Design review of the part built by this model. Coordinates are the model's own, in mm. A direction names the side the tool comes from. Coordinates: 2 decimals unless noted, no trailing zeros. Order: outer loops, then holes, each group sorted by start corner. A loop starts at its lowest first (then second) coordinate and runs counter-clockwise, first axis right, second up. Notation, with made-up numbers: M 28,59.5 L 77,59.5 A18 ccw 77,70.5 Z; hole C 74,-23 d7. An arc over 180 degrees is marked long. Answer as a JSON object with one key per item and string values.
from build123d import *

# Parameters (mm, degrees)
SKETCH3_R           = 12.7
BOSS_EXTRUDE1_DEPTH = 381
SKETCH4_W           = 50.8
SKETCH4_H           = 50.8
BOSS_EXTRUDE2_DEPTH = 25.4
SKETCH5_W           = 50.8
SKETCH5_H           = 50.8
BOSS_EXTRUDE3_DEPTH = 25.4
SKETCH6_R           = 1.016
SKETCH6_R_2         = 0.9921875
CUT_EXTRUDE1_DEPTH  = 411.349558304


with BuildPart() as part:
    # Sketch3 → Boss-Extrude1 (new body)
    with BuildSketch(Plane.XY):
        Circle(SKETCH3_R)
    extrude(amount=BOSS_EXTRUDE1_DEPTH)

    # Sketch4 → Boss-Extrude2 (add, symmetric)
    with BuildSketch(Plane(origin=(0, 0, 0), x_dir=(-1, 0, 0), z_dir=(0, 0, -1))):
        Rectangle(SKETCH4_W, SKETCH4_H)
    extrude(amount=BOSS_EXTRUDE2_DEPTH, both=True)

    # Sketch5 → Boss-Extrude3 (add, symmetric)
    with BuildSketch(Plane.XY.offset(381)):
        Rectangle(SKETCH5_W, SKETCH5_H)
    extrude(amount=BOSS_EXTRUDE3_DEPTH, both=True)

    # Sketch6 → Cut-Extrude1 (cut, through all)
    with BuildSketch(Plane(origin=(0, 25.4, 0), x_dir=(1, 0, 0), z_dir=(0, 1, 0))):
        with Locations(Location((0, -381, 0), (0, 0, 270))):
            Circle(SKETCH6_R)
        with Locations(Location((0, 0, 0), (0, 0, 270))):
            Circle(SKETCH6_R_2)
    extrude(amount=-CUT_EXTRUDE1_DEPTH, mode=Mode.SUBTRACT)


solid = part.part
1) Add section B-B (z = 326). State the section outline as (x, y) points, and give its area (3 significant figures).
Taken from the geometry:
{"outline": "C 0,0 d25.4", "area": "507 mm2"}
2) Add section A-A (y = 0). State the section outline as (x, z) points, and give its area (3 significant figures).
Taken from the geometry:
{"outline": "M -25.4,-25.4 L 25.4,-25.4 L 25.4,25.4 L 12.7,25.4 L 12.7,355.6 L 25.4,355.6 L 25.4,406.4 L -25.4,406.4 L -25.4,355.6 L -12.7,355.6 L -12.7,25.4 L -25.4,25.4 Z; hole C 0,381 d2.03; hole C 0,0 d1.98", "area": "13,500 mm2"}
3) To check wall thickness, follow L1, parallel to Z at x = -3, y = 17.5; L2, parallel to X at y = 9, z = 381; L3, parallel to Y at x = -0.5, z = 234. State the ranges of each line that lie inside material, in increasing order.
Taken from the geometry:
{"L1": "z = -25.4 to 25.4, 355.6 to 406.4", "L2": "x = -25.4 to -1.02, 1.02 to 25.4", "L3": "y = -12.69 to 12.69"}
4) Add section C-C (x = 7.5). State the section outline as (y, z) points.
Taken from the geometry:
{"outline": "M -25.4,-25.4 L 25.4,-25.4 L 25.4,25.4 L 10.25,25.4 L 10.25,355.6 L 25.4,355.6 L 25.4,406.4 L -25.4,406.4 L -25.4,355.6 L -10.25,355.6 L -10.25,25.4 L -25.4,25.4 Z"}
5) Tool access review of faces 1 (the flat face through (-5, -25.4, 0)), 2 (the flat face through (6, 12, 25.4)): name each direction out of +Z, -Z, +X, -X, +Y, -Y from which nothing blocks a thin tool from reaching the whole face with its end or side.
Taken from the geometry:
{"face 1": "+Z, -Z, +X, -X, -Y", "face 2": "none"}
6) Insertion check: pin 1 Ø4 at (y, z) = (2, 166) entering from -X; pin 2 Ø3 at (x, z) = (9.5, 90.5) entering from -Y; pin 3 Ø3 at (x, z) = (0, 78.5) entering from +Y. Each pin has a flat end and moves straight along its axis. Give the tip position at first contact, or say it passes through.
Taken from the geometry:
{"pin 1": "stops at x = -12.7", "pin 2": "stops at y = -9.86", "pin 3": "stops at y = 12.7"}
